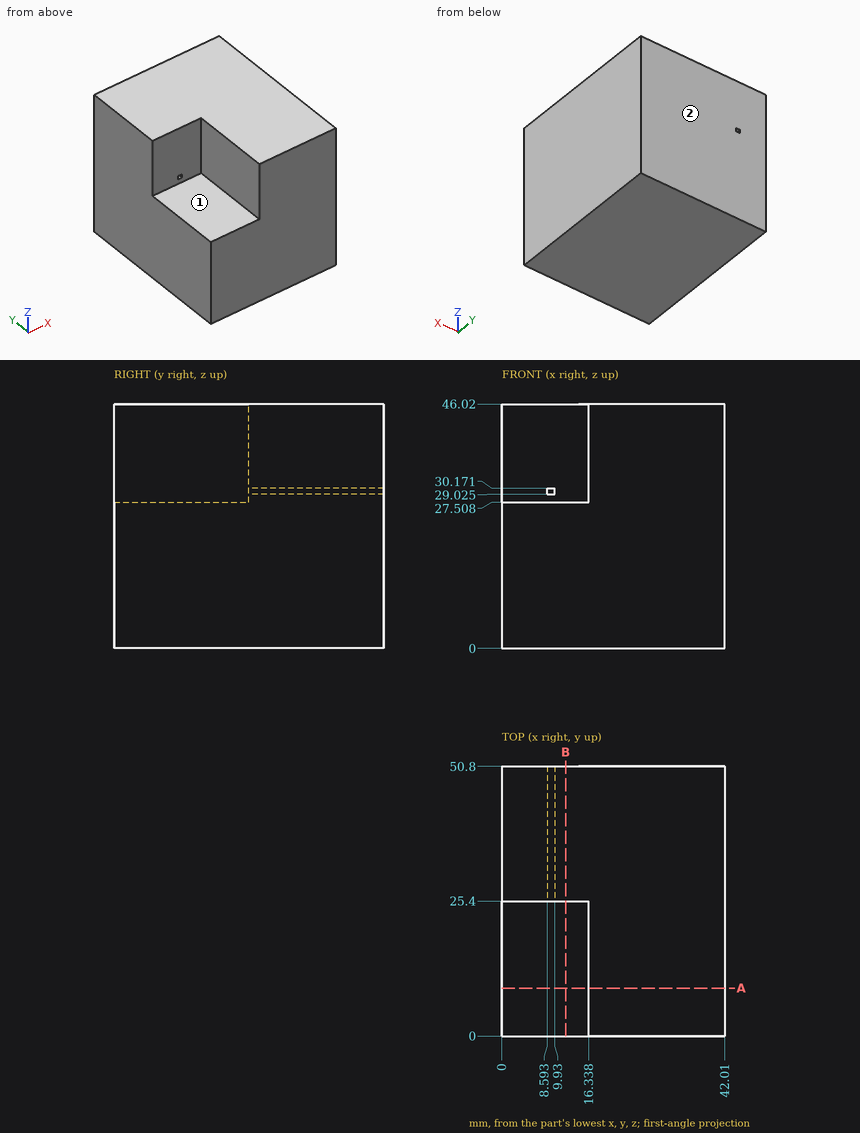
Part print with two shaded views. Sizes in mm from the minimum x, y, z corner. A direction names the side the tool comes from. Coordinates: 2 decimals unless noted, no trailing zeros. Order: outer loops, then holes, each group sorted by start corner. A loop starts at its lowest first (then second) coordinate and runs counter-clockwise, first axis right, second up. Notation, with made-up numbers: M 80,19 L 109,19 A25 cw 109,43 Z; hole C 68.25,7 d3. An arc over 180 degrees is marked long. One line per question, with ' | ' between items. Start each with the question number.
1. Wall check: line 1 along X through (y, z) = (14, 33.5); line 2 along Z through (x, y) = (2, 22.5). Give the ranges that are in metal, low to high. Write a range as [from, to].
2. Cut at A-A (y = 9). Write the cut outline in (x, z), plus the area to 3 significant figures.
3. Cut at B-B (x = 12). Write the cut outline in (y, z), plus the area to 3 significant figures.
4. Flat gauge pins, fed straight in: P1, Ø4, axis at x = 9, y = 8.5, coming from the +Z side; P2, Ø15, axis at y = 17, z = 36, coming from the -X side; P3, Ø5, axis at x = 10.5, z = 38.5, coming from the -Y side. Where does each tip first touch, or does it go through?
5. Tool access for the marked faces 1 and 2: list every direction of +Z, -Z, +X, -X, +Y, -Y with a clear straight run to the whole face (end or side of a thin tool).
The answers:
1) line 1: x = [16.34, 42.01] | line 2: z = [0, 27.51]
2) outline: M 0,0 L 42.01,0 L 42.01,46.02 L 16.34,46.02 L 16.34,27.51 L 0,27.51 Z | area: 1,630 mm2
3) outline: M 0,0 L 50.8,0 L 50.8,46.02 L 25.4,46.02 L 25.4,27.51 L 0,27.51 Z | area: 1,870 mm2
4) P1: stops at z = 27.51 | P2: stops at x = 16.34 | P3: stops at y = 25.4
5) face 1: +Z, -X, -Y | face 2: +Z, -Z, +X, -X, +Y
